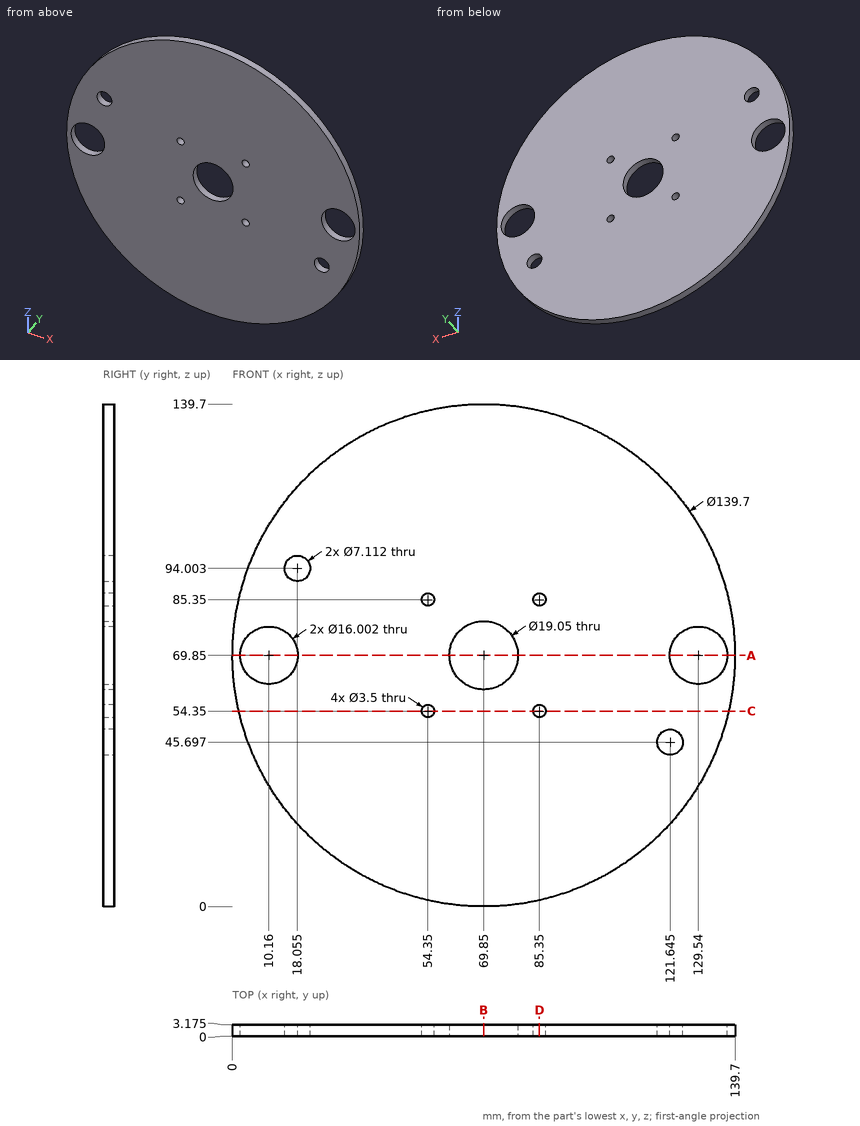
Study the drawing (mm; zero at the part's minimum x, y, z) and answer. Round coordinates to 2 decimals unless told otherwise and drop trailing zeros. Write each loop counter-clockwise with the first axis right and the second up, starting at its lowest first coordinate (ties: lowest second). Pieces come first, ordered by that corner, then holes. Notation, with made-up numbers: (-23.75, 88) -> (30.25, 88) arc R26 cw to (30.25, 116) -> close; hole circle Ø1 at (7.25, 69). An arc over 180 degrees is marked (long way). Write each question's results on one line, items separated by ' | '.
Item 1: A flat-ended cylindrical pin translates along its axis: P1, Ø2, axis at x = 85.35, z = 85.35, coming from the +Y side. Find the tip coordinate at first contact, or state that the pin passes through.
Result set:
P1: through
Item 2: A cutting plane is placed at B-B, the plane x = 69.85. Determine the outline of the cut face in (y, z) (1 decimal).
Result set:
outline: (0, 0) -> (3.2, 0) -> (3.2, 60.3) -> (0, 60.3) -> close; (0, 79.4) -> (3.2, 79.4) -> (3.2, 139.7) -> (0, 139.7) -> close
Item 3: Find the intervals of material crossed by line 1 along X through (y, z) = (0.9, 69.85) (1 decimal); line 2 along Z through (x, y) = (54.35, 0.75); line 3 along Z through (x, y) = (70.5, 2.7), in increasing order. Write a range as [from, to].
Result set:
line 1: [0, 2.2], [18.2, 60.3], [79.4, 121.5], [137.5, 139.7] | line 2: [1.74, 52.6], [56.1, 83.6], [87.1, 137.96] | line 3: [0, 60.35], [79.35, 139.7]
Item 4: A cutting plane is placed at C-C, the plane z = 54.35. Determine the outline of the cut face in (x, y) (1 decimal).
Result set:
outline: (1.7, 0) -> (52.6, 0) -> (52.6, 3.2) -> (1.7, 3.2) -> close; (56.1, 0) -> (83.6, 0) -> (83.6, 3.2) -> (56.1, 3.2) -> close; (87.1, 0) -> (138, 0) -> (138, 3.2) -> (87.1, 3.2) -> close
Item 5: A cutting plane is placed at D-D, the plane x = 85.35. Determine the outline of the cut face in (y, z) (1 decimal).
Result set:
outline: (0, 1.7) -> (3.2, 1.7) -> (3.2, 52.6) -> (0, 52.6) -> close; (0, 56.1) -> (3.2, 56.1) -> (3.2, 83.6) -> (0, 83.6) -> close; (0, 87.1) -> (3.2, 87.1) -> (3.2, 138) -> (0, 138) -> close
Item 6: A cutting plane is placed at A-A, the plane z = 69.85. Determine the outline of the cut face in (x, y) (1 decimal).
Result set:
outline: (0, 0) -> (2.2, 0) -> (2.2, 3.2) -> (0, 3.2) -> close; (18.2, 0) -> (60.3, 0) -> (60.3, 3.2) -> (18.2, 3.2) -> close; (79.4, 0) -> (121.5, 0) -> (121.5, 3.2) -> (79.4, 3.2) -> close; (137.5, 0) -> (139.7, 0) -> (139.7, 3.2) -> (137.5, 3.2) -> close
